from build123d import *

# Parameters (mm, degrees)
SKETCH1_W               = 25.4
SKETCH1_H               = 5.08
BOSS_EXTRUDE1_DEPTH     = 2
SKETCH2_W               = 3
SKETCH2_H               = 5.08
BOSS_EXTRUDE2_DEPTH     = 27
SKETCH3_R               = 1.5
BOSS_EXTRUDE3_DEPTH     = 5.08
CUT_EXTRUDE1_DEPTH      = 39.634331882
CUT_EXTRUDE1_DEPTH_BACK = 39.634331882
SKETCH4_W               = 3.08
SKETCH4_H               = 28


with BuildPart() as part:
    # Sketch1 → Boss-Extrude1 (new body)
    with BuildSketch(Plane(origin=(0, 0, 0), x_dir=(1, 0, 0), z_dir=(0, 1, 0))):
        Rectangle(SKETCH1_W, SKETCH1_H)
    extrude(amount=BOSS_EXTRUDE1_DEPTH)

    # Sketch2 → Boss-Extrude2 (add)
    with BuildSketch(Plane(origin=(0, 2, 0), x_dir=(1, 0, 0), z_dir=(0, 1, 0))):
        with Locations((11.2, 0)):
            Rectangle(SKETCH2_W, SKETCH2_H)
    boss_extrude2 = extrude(amount=BOSS_EXTRUDE2_DEPTH)

    # Sketch3 → Boss-Extrude3 (add)
    with BuildSketch(Plane.ZY.offset(-9.7)):
        with Locations((1.04, 27.5)):
            Circle(SKETCH3_R)
    boss_extrude3 = extrude(amount=BOSS_EXTRUDE3_DEPTH)

    # Mirror1: Boss-Extrude2, Boss-Extrude3 across plane
    add(boss_extrude2.mirror(Plane(origin=(0, 0, 0), x_dir=(0, 0, 1), z_dir=(1, 0, 0))))
    add(boss_extrude3.mirror(Plane(origin=(0, 0, 0), x_dir=(0, 0, 1), z_dir=(1, 0, 0))))

    # Sketch4 → Cut-Extrude1 (cut, two sides: drawn at the far end of the back side and taken through both)
    with BuildSketch(Plane.ZY.offset(12.7).offset(-CUT_EXTRUDE1_DEPTH_BACK)):
        with Locations((0, 14)):
            Rectangle(SKETCH4_W, SKETCH4_H)
    extrude(amount=CUT_EXTRUDE1_DEPTH + CUT_EXTRUDE1_DEPTH_BACK, mode=Mode.SUBTRACT)


solid = part.part
Source: CAD feature listing. Evaluate the final solid. Frame: model axes, mm. A direction names the side the tool comes from. Round coordinates to 2 decimals unless told otherwise and drop trailing zeros. Write each loop counter-clockwise with the first axis right and the second up, starting at its lowest first coordinate (ties: lowest second). Pieces come first, ordered by that corner, then holes. Notation, with made-up numbers: M -24.5,88 L -8.5,88 A33 cw -8.5,125 Z; hole C 59.25,82 d2. An arc over 180 degrees is marked long. One line per item, written item: value. Start each with the question number.
Item 1: Ray query, L1, parallel to X at y = 11.5, z = 2; L2, parallel to Z at x = -10.5, y = 14.75; L3, parallel to Y at x = -8.5, z = 1.9. Return the intervals inside material, ascending. Write a range as from..to.
Item 2: Section query C-C (y = 4.25). Return the cut outline in (x, z), plus the area to 3 significant figures.
Item 3: Section query B-B (z = -0.9). Return the cut outline in (x, y).
Item 4: Section query A-A (x = -5.5). Return the cut outline in (y, z).
Item 5: Set-up query: faces 1 (the flat face through (-9, 28, 0)), 2 (the flat face through (0, 2, -2)), 3 (the flat face through (0, 2, 2)), 4 (the flat face through (9.7, 15, -2)), 5 (the flat face through (-9.7, 28.64, 2.24)). Return all of +Z, -Z, +X, -X, +Y, -Y with unobstructed straight access to the full face (end or side cutting, diameter ignored); none if empty.
Item 6: Mould query, pull axis Y, two halves, no side actions, for faces 6 (the cylindrical face through (7.2, 28.53, 2.13)), 7 (the flat face through (0, 0, -2)), 8 (the flat face through (4.62, 28, 2)), 9 (the flat face through (9.7, 15, 2)). Classes: pulls with the +Y half, pulls with the -Y half, needs draft (parallel to the pull), parting line crosses it, or undercut.
Item 7: Section query D-D (x = -2). Return the cut outline in (y, z), plus the area to 3 significant figures.
Item 8: Pin query (flat end, axial travel): pin 1 (12 mm diameter, centred on x = -6, y = 25, fed in from -Z); pin 2 (1.8 mm diameter, centred on y = 10.5, z = -0.5, fed in from -X); pin 3 (1.5 mm diameter, centred on x = 8.5, z = 0.5, fed in from -Y). Return the tip coordinate at first contact, or that it passes through.
Result set:
1. L1: x = -12.7..-9.7, 9.7..12.7
1. L2: z = -2.54..-1.54, 1.54..2.54
1. L3: y = 0..2, 26.27..28.73
2. outline: M -12.7,-2.54 L -9.7,-2.54 L -9.7,-1.54 L -12.7,-1.54 Z; M -12.7,1.54 L -9.7,1.54 L -9.7,2.54 L -12.7,2.54 Z; M 9.7,-2.54 L 12.7,-2.54 L 12.7,-1.54 L 9.7,-1.54 Z; M 9.7,1.54 L 12.7,1.54 L 12.7,2.54 L 9.7,2.54 Z
2. area: 12.0 mm²
3. outline: M -12.7,28 L -9.7,28 L -9.7,29 L -12.7,29 Z; M 9.7,28 L 12.7,28 L 12.7,29 L 9.7,29 Z
4. outline: M 0,-2.54 L 2,-2.54 L 2,-1.54 L 0,-1.54 Z; M 0,1.54 L 2,1.54 L 2,2.54 L 0,2.54 Z; M 26.09,1.54 L 28,1.54 L 28,-0.37 A1.5 ccw long Z
5. face 1: +X, -X, -Y
5. face 2: +Z, -Z, +Y
5. face 3: +Z, -Z
5. face 4: -Z, +Y
5. face 5: +Z, +Y
6. face 6: undercut
6. face 7: pulls with the -Y half
6. face 8: needs draft
6. face 9: undercut
7. outline: M 0,-2.54 L 2,-2.54 L 2,-1.54 L 0,-1.54 Z; M 0,1.54 L 2,1.54 L 2,2.54 L 0,2.54 Z
7. area: 4.00 mm²
8. pin 1: stops at z = -2.54
8. pin 2: passes through
8. pin 3: stops at y = 28
